Could you check a few things on this drawing? It's one solid part, dimensions in mm from its lowest x, y, z. A direction names the side the tool comes from. Coordinates: 2 decimals unless noted, no trailing zeros. Write each loop counter-clockwise with the first axis right and the second up, starting at its lowest first coordinate (ties: lowest second). Pieces come first, ordered by that corner, then holes. Notation, with made-up numbers: (43.25, 57) - (90.25, 57) arc R13 ccw to (90.25, 81) - close; hole circle Ø8 at (65.5, -33.5). An arc over 180 degrees is marked (long way). Answer as a JSON object with one key per item and string values. Group by question number.
1) If we section it at D-D (x = 19.75): Write out the boundary of the cut face in (y, z) (1 decimal), plus the area to 3 significant figures.
2) If we section it at B-B (x = 12.5): Write out the boundary of the cut face in (y, z).
3) On a 3-axis mill with a long thin cutter (end or side, diameter ignored), from which of +Z, -Z, +X, -X, +Y, -Y can I reach the whole of each face in a straight line? I mean the marked faces 1 and 2. Say none if no direction works.
4) Please list where these lines run through material, in increasing order: line 1 along X through (y, z) = (9.55, 12.5); line 2 along Z through (x, y) = (7.5, 2) (1 decimal); line 3 along Y through (x, z) = (20.25, 7.25).
5) We'd pull the mould along Z, two halves only. Please class the marked faces 3, 4, 5 and 6: released by +Z, released by -Z, zero draft, split by the parting line, or undercut.
6) If we section it at C-C (z = 12.5): Write out the boundary of the cut face in (x, y).
7) Will these pins go through, and if not, where does the flat tip stop? pin 1 Ø4 at (y, z) = (8.5, 11) entering from +X; pin 2 Ø4.5 at (x, z) = (6.49, 6.49) entering from +Y; pin 3 Ø1.5 at (x, z) = (12.5, 13.5) entering from +Y; pin 4 Ø3 at (x, z) = (6.49, 18.51) entering from -Y.
8) If we section it at A-A (z = 5.75): Write out the boundary of the cut face in (x, y) (1 decimal).
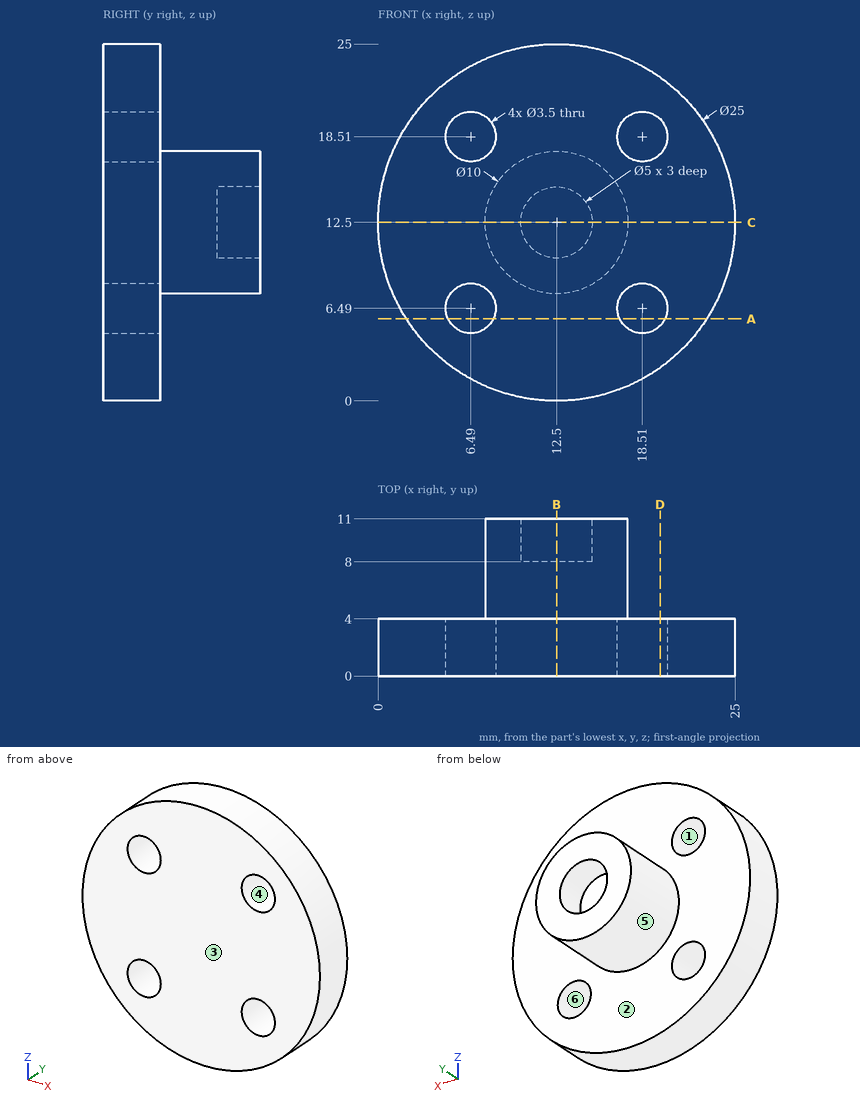
Here are the results:
{
 "1": {"outline": "(0, 2.3) - (4, 2.3) - (4, 5.3) - (0, 5.3) - close; (0, 7.7) - (4, 7.7) - (4, 17.3) - (0, 17.3) - close; (0, 19.7) - (4, 19.7) - (4, 22.7) - (0, 22.7) - close", "area": "61.7 mm²"},
 "2": {"outline": "(0, 0) - (4, 0) - (4, 7.5) - (11, 7.5) - (11, 10) - (8, 10) - (8, 15) - (11, 15) - (11, 17.5) - (4, 17.5) - (4, 25) - (0, 25) - close"},
 "3": {"face 1": "+Y, -Y", "face 2": "+Y"},
 "4": {"line 1": "x = 7.5 to 10, 15 to 17.5", "line 2": "z = 1 to 5.1, 7.9 to 17.1, 19.9 to 24", "line 3": "y = 0 to 4"},
 "5": {"face 3": "zero draft", "face 4": "undercut", "face 5": "split by the parting line", "face 6": "undercut"},
 "6": {"outline": "(0, 0) - (25, 0) - (25, 4) - (17.5, 4) - (17.5, 11) - (15, 11) - (15, 8) - (10, 8) - (10, 11) - (7.5, 11) - (7.5, 4) - (0, 4) - close"},
 "7": {"pin 1": "stops at x = 17.5", "pin 2": "stops at y = 4", "pin 3": "stops at y = 8", "pin 4": "passes through"},
 "8": {"outline": "(2, 0) - (4.9, 0) - (4.9, 4) - (2, 4) - close; (8.1, 0) - (16.9, 0) - (16.9, 4) - (8.1, 4) - close; (20.1, 0) - (23, 0) - (23, 4) - (20.1, 4) - close"}
}
